The model under review builds one solid part; all positions refer to its coordinate system, in mm. Face numbers are marked on the shaded views. A direction names the side the tool comes from. Coordinates: 2 decimals unless noted, no trailing zeros. Write each loop counter-clockwise with the first axis right and the second up, starting at its lowest first coordinate (ties: lowest second). Pieces come first, ordered by that corner, then holes.
1) Machinability: for the marked faces 1 and 2, which of the approach directions +Z, -Z, +X, -X, +Y, -Y give a long, thin tool a straight path to every point of the face, cutting with its end or side? Answer none if there is none.
2) Add section C-C, the plane x = 26. State the section outline as (y, z) points, then the cut area to 3 significant figures.
3) For line 1 (Y direction, x = 18.5, z = 0); line 2 (Y direction, x = 37, z = 0); line 3 (Z direction, x = 8.5, y = 13), list the stretches that pass through material, from the lowest coordinate up.
4) For P1, Ø8, axis at x = 7.5, z = 2.5, coming from the +Y side; P2, Ø10, axis at x = 27, y = -8, coming from the -Z side; P3, Ø1, axis at y = -7, z = 11, coming from the -X side, all flat-tipped, find the tip position at first contact; note any pin that passes through.
5) Add section A-A, the plane y = 0. State the section outline as (x, z) points, then the cut area to 3 significant figures.
6) Mouldability with a two-part tool opening along Z and no side actions: class the marked faces 3, 4 and 5 as released by +Z, released by -Z, zero draft, split by the parting line, or undercut.
7) Add section D-D, the plane x = 4.5. State the section outline as (y, z) points, then the cut area to 3 significant figures.
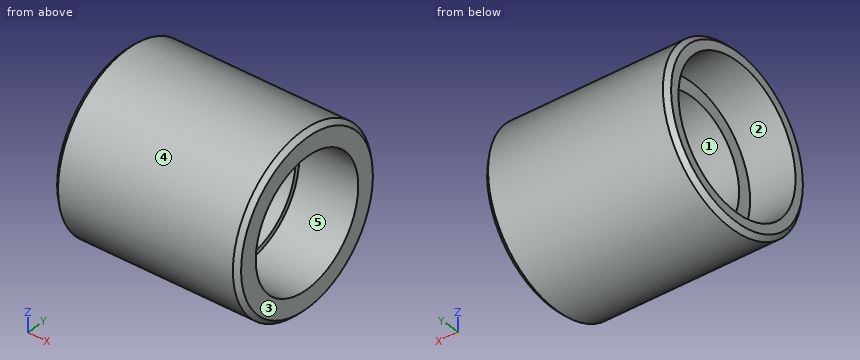
from build123d import *


with BuildPart() as part:
    # Esquisse1 → Base-Révolution (revolve)
    with BuildSketch(Plane.XY, mode=Mode.PRIVATE) as base_r_volution_sk:
        Polygon((0, 18), (0, 16), (10, 16), (10, 13), (27.5, 13), (27.5, 14), (40.5, 14), (40.5, 18), (39.5, 19), (1, 19), align=None)
    revolve(base_r_volution_sk.sketch.rotate(Axis((0, 0, 0), (1, 0, 0)), 90), axis=Axis((0, 0, 0), (1, 0, 0)))


solid = part.part
Geometry results:
1. face 1: +X, -X
1. face 2: -X
2. outline: circle Ø38 at (0, 0); hole circle Ø26 at (0, 0)
2. area: 603 mm2
3. line 1: y = -19 to -13, 13 to 19
3. line 2: y = -19 to -14, 14 to 19
3. line 3: z = -13.86 to -9.33, 9.33 to 13.86
4. P1: stops at y = 19
4. P2: stops at z = -18.76
4. P3: stops at x = 10
5. outline: (0, -18) - (1, -19) - (39.5, -19) - (40.5, -18) - (40.5, -14) - (27.5, -14) - (27.5, -13) - (10, -13) - (10, -16) - (0, -16) - close; (0, 16) - (10, 16) - (10, 13) - (27.5, 13) - (27.5, 14) - (40.5, 14) - (40.5, 18) - (39.5, 19) - (1, 19) - (0, 18) - close
5. area: 398 mm2
6. face 3: zero draft
6. face 4: split by the parting line
6. face 5: undercut
7. outline: circle Ø38 at (0, 0); hole circle Ø32 at (0, 0)
7. area: 330 mm2
